```python
from build123d import *
from OCP.BRepFilletAPI import BRepFilletAPI_MakeChamfer

# Parameters (mm, degrees)
BOSS_EXTRU_1_DEPTH           = 70
BOSS_EXTRU_1_DEPTH_BACK      = 70
ESQUISSE12_W                 = 129.6
ESQUISSE12_H                 = 246.867117592
BOSS_EXTRU_7_DEPTH           = 1.5
CHANFREIN1_SIZE              = 1.5
CHANFREIN1_SIZE_2            = 1.787630389
ENL_V_MAT_EXTRU_1_DEPTH      = 209.036677197
ENL_V_MAT_EXTRU_1_DEPTH_BACK = 209.036677197
BOSS_EXTRU_4_START           = -10
ESQUISSE5_R                  = 1.9
BOSS_EXTRU_4_DEPTH           = 10
ENL_V_MAT_EXTRU_2_DEPTH      = 146.364588204
ENL_V_MAT_EXTRU_2_DEPTH_BACK = 146.364588204
ESQUISSE6_W                  = 22.24
ESQUISSE6_H                  = 15
ESQUISSE7_W                  = 22.24
ESQUISSE7_H                  = 10
BOSS_EXTRU_5_DEPTH           = 10
ESQUISSE8_R                  = 1.25
ENL_V_MAT_EXTRU_3_DEPTH      = 229.570143353
BOSS_EXTRU_6_DEPTH           = 20
ENL_V_MAT_EXTRU_4_DEPTH      = 147.654246266
ENL_V_MAT_EXTRU_4_DEPTH_BACK = 147.654246266
ESQUISSE11_R                 = 1.5


with BuildPart() as part:
    # Esquisse1 → Boss.-Extru.1 (new, two sides: drawn at the far end of the back side and taken through both)
    with BuildSketch(Plane(origin=(0, 0, 0), x_dir=(0, -1, 0), z_dir=(1, 0, 0)).offset(-BOSS_EXTRU_1_DEPTH_BACK)):
        Polygon((0, -123.433558796), (0, 123.433558796), (-3.830222216, 126.647496845), (-3.830222216, -126.647496845), align=None)
    extrude(amount=BOSS_EXTRU_1_DEPTH + BOSS_EXTRU_1_DEPTH_BACK)

    # Esquisse12 → Boss.-Extru.7 (add)
    with BuildSketch(Plane(origin=(0, 0, 0), x_dir=(-1, 0, 0), z_dir=(0, -1, 0))):
        Rectangle(ESQUISSE12_W, ESQUISSE12_H)
    extrude(amount=BOSS_EXTRU_7_DEPTH)

    # Chanfrein1
    chanfrein1_edges_1 = [part.edges().sort_by_distance(p)[0] for p in [
        (0, -1.5, 123.433558796),
    ]]
    chanfrein1_side_1 = [part.faces().sort_by_distance(p)[0] for p in [
        (0, -1.47, 123.433558796),
    ]]
    chanfrein1_edges_2 = [part.edges().sort_by_distance(p)[0] for p in [
        (0, -1.5, -123.433558796),
    ]]
    chanfrein1_side_2 = [part.faces().sort_by_distance(p)[0] for p in [
        (0, -1.47, -123.433558796),
    ]]
    chanfrein1 = BRepFilletAPI_MakeChamfer(part.part.solid().wrapped)
    for e in chanfrein1_edges_1:
        chanfrein1.Add(CHANFREIN1_SIZE - 0.0001, CHANFREIN1_SIZE_2 - 0.0001, e.wrapped, chanfrein1_side_1[0].wrapped)
    for e in chanfrein1_edges_2:
        chanfrein1.Add(CHANFREIN1_SIZE - 0.0001, CHANFREIN1_SIZE_2 - 0.0001, e.wrapped, chanfrein1_side_2[0].wrapped)
    add(Compound.cast(chanfrein1.Shape()), mode=Mode.REPLACE)  # a hair under: the kernel refuses the full size

    # Esquisse4 → Enlèv. mat.-Extru.1 (cut, two sides: drawn at the far end of the back side and taken through both)
    with BuildSketch(Plane(origin=(95, 0, 0), x_dir=(-1, 0, 0), z_dir=(0, -1, 0)).offset(-ENL_V_MAT_EXTRU_1_DEPTH_BACK)):
        with BuildLine():
            Line((105, -25.151970252), (85, -25.151970252))
            Line((85, -25.151970252), (85, -10.151970252))
            ThreePointArc((85, -10.151970252), (95, 14.25), (105, -10.151970252))
            Line((105, -10.151970252), (105, -25.151970252))
        make_face()
    extrude(amount=ENL_V_MAT_EXTRU_1_DEPTH + ENL_V_MAT_EXTRU_1_DEPTH_BACK, mode=Mode.SUBTRACT)

    # Esquisse5 → Boss.-Extru.4 (add)
    with BuildSketch(Plane(origin=(95, 3.830222216, 0), x_dir=(-1, 0, 0), z_dir=(0, -1, 0)).offset(BOSS_EXTRU_4_START)):
        with BuildLine():
            Line((105, -10.151970252), (111.823043033, -10.151970252))
            ThreePointArc((111.823043033, -10.151970252), (113.951535544, -9.489367154), (115.327843665, -7.735714055))
            ThreePointArc((115.327843665, -7.735714055), (95, 21.75), (74.672156335, -7.735714055))
            ThreePointArc((74.672156335, -7.735714055), (76.048464456, -9.489367154), (78.176956967, -10.151970252))
            Line((78.176956967, -10.151970252), (85, -10.151970252))
            ThreePointArc((85, -10.151970252), (95, 14.25), (105, -10.151970252))
        make_face()
        with Locations(Location((77.5, 0, 0), (0, 0, 90))):
            Circle(ESQUISSE5_R, mode=Mode.SUBTRACT)
        with Locations(Location((112.5, 0, 0), (0, 0, 90))):
            Circle(ESQUISSE5_R, mode=Mode.SUBTRACT)
    extrude(amount=BOSS_EXTRU_4_DEPTH)

    # Esquisse6 → Enlèv. mat.-Extru.2 (cut, two sides: drawn at the far end of the back side and taken through both)
    with BuildSketch(Plane(origin=(0, 0, 0), x_dir=(-1, 0, 0), z_dir=(0, -1, 0)).offset(-ENL_V_MAT_EXTRU_2_DEPTH_BACK)):
        with Locations((0, 83)):
            Rectangle(ESQUISSE6_W, ESQUISSE6_H)
    extrude(amount=ENL_V_MAT_EXTRU_2_DEPTH + ENL_V_MAT_EXTRU_2_DEPTH_BACK, mode=Mode.SUBTRACT)

    # Esquisse7 → Boss.-Extru.5 (add)
    with BuildSketch(Plane(origin=(0, 3.830222216, 0), x_dir=(1, 0, 0), z_dir=(0, 1, 0))):
        with Locations((0, 95.5)):
            Rectangle(ESQUISSE7_W, ESQUISSE7_H)
    extrude(amount=BOSS_EXTRU_5_DEPTH)

    # Esquisse8 → Enlèv. mat.-Extru.3 (cut, through all)
    with BuildSketch(Plane.XY.offset(-90.5)):
        with Locations((-8.02, 10.830222216)):
            Circle(ESQUISSE8_R)
        with Locations((8.02, 10.830222216)):
            Circle(ESQUISSE8_R)
    extrude(amount=-ENL_V_MAT_EXTRU_3_DEPTH, mode=Mode.SUBTRACT)

    # Esquisse9 → Boss.-Extru.6 (add)
    with BuildSketch(Plane(origin=(0, 3.830222216, 0), x_dir=(1, 0, 0), z_dir=(0, 1, 0))):
        Polygon((-14.5, 114.647496845), (14.5, 114.647496845), (14.5, 126.647496845), (16.5, 126.647496845), (16.5, 109.647496845), (-16.5, 109.647496845), (-16.5, 126.647496845), (-14.5, 126.647496845), align=None)
    extrude(amount=BOSS_EXTRU_6_DEPTH)

    # Esquisse11 → Enlèv. mat.-Extru.4 (cut, two sides: drawn at the far end of the back side and taken through both)
    with BuildSketch(Plane(origin=(0, 0, 0), x_dir=(0, 0, -1), z_dir=(1, 0, 0)).offset(-ENL_V_MAT_EXTRU_4_DEPTH_BACK)):
        with Locations((121.647496845, 18.830222216)):
            Circle(ESQUISSE11_R)
    extrude(amount=ENL_V_MAT_EXTRU_4_DEPTH + ENL_V_MAT_EXTRU_4_DEPTH_BACK, mode=Mode.SUBTRACT)


solid = part.part
```
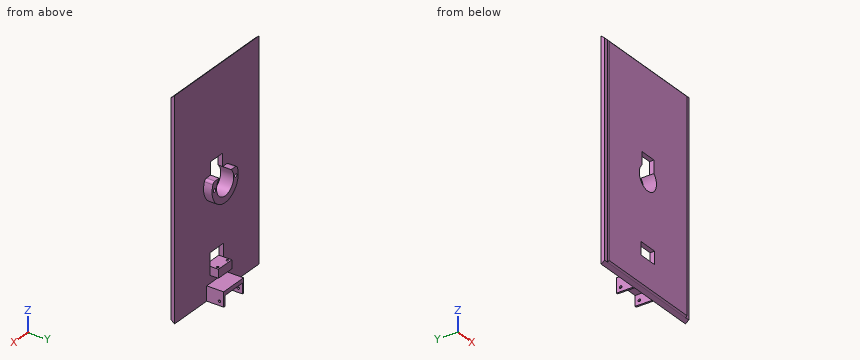
For this review, take the finished solid that the model builds, in its own axes (mm). Round coordinates to 2 decimals unless told otherwise and drop trailing zeros. Write each loop counter-clockwise with the first axis right and the second up, starting at its lowest first coordinate (ties: lowest second). Pieces come first, ordered by that corner, then holes. Notation, with made-up numbers: (-3, -5.75) -> (38, -5.75) arc R34 ccw to (38, 33.25) -> close; hole circle Ø8 at (-24, 58.5). An arc over 180 degrees is marked (long way). Use one line per item in the form item = value.
1) To check wall thickness, follow L1, parallel to X at y = 7, z = 0; L2, parallel to Y at x = 8.02, z = -93.25; L3, parallel to X at y = 10, z = -93. State the ranges of each line that lie inside material, in increasing order. Write a range as from..to.
Found:
L1 = -21.75..-19.4, -15.6..-14.25, 14.25..15.6, 19.4..21.75
L2 = -1.5..9.58, 12.08..13.83
L3 = -11.12..-8.95, -7.09..7.09, 8.95..11.12
2) Take a section at A-A, the plane x = 0. Count the separate pieces of the cut face and the enclosed holes in it, and give its area (3 significant figures).
Found:
separate_pieces = 3
enclosed_holes = 0
area = 1,310 mm2
3) Clearance check with flat-ended pins moving along their axes: pin 1 (3.5 mm diameter, centred on y = 18.83, z = -121.65, fed in from -X); pin 2 (1.6 mm diameter, centred on x = -0.5, y = 0.5, fed in from -Z); pin 3 (12.5 mm diameter, centred on x = -2, y = 6.5, fed in from +Z); pin 4 (23 mm diameter, centred on x = 0, z = 0, fed in from -Y). State where each tip first meets the part, or that it passes through.
Found:
pin_1 = -16.5
pin_2 = -124.52
pin_3 = 126.65
pin_4 = through
4) Take a section at C-C, the plane z = 33. Write out the cut boundary in (x, y).
Found:
outline = (-70, 0) -> (-64.8, 0) -> (-64.8, -1.5) -> (64.8, -1.5) -> (64.8, 0) -> (70, 0) -> (70, 3.83) -> (-70, 3.83) -> close
